Autodesk Inventor part; units mm, degrees
ref_plane "YZ Plane" through (0, 0, 0) normal (1, 0, 0) x (0, 1, 0)
ref_plane "XZ Plane" through (0, 0, 0) normal (0, 1, 0) x (-1, 0, 0)
ref_plane "XY Plane" through (0, 0, 0) normal (0, 0, 1) x (1, 0, 0)
sketch "Sketch1" plane through (0, 0, 0) normal (0, 0, 1) x (1, 0, 0)
  line L0 (-9.4319, 10.8445) -> (26.5681, 10.8445)
  line L1 (26.5681, 10.8445) -> (26.5681, -46.1555)
  line L2 (26.5681, -46.1555) -> (-9.4319, -46.1555)
  line L3 (-9.4319, -46.1555) -> (-9.4319, 10.8445)
  point P0 (0, 0)
  dimension "d0" = 36
  dimension "d1" = 57
extrude "Extrusion1" add sketch "Sketch1" along normal blind 3
sketch "Sketch2" plane through (-9.4319, 10.8445, 0) normal (0, 1, 0) x (1, 0, 0)
  line L0 (0, 0) -> (36, 0) construction
  line L1 (0, -3) -> (0, -22.268)
  line L2 (36, -3) -> (36, -22.268)
  line L3 (18, 0) -> (18, -6.949) construction
  arc A0 (36, -22.268) -> (0, -22.268) centre (18, -25.1836) ccw
  line L4 (36, -3) -> (0, -3)
  line L5 (36, -3) -> (0, -3)
  point P0 (9.4319, 0)
  dimension "d4" = 22.268
  dimension "d5" = 6.949
extrude "Extrusion2" add sketch "Sketch2" against normal blind 3
sketch "Sketch3" plane through (-9.4319, -46.1555, 0) normal (0, -1, 0) x (1, 0, 0)
  line L0 (0, 0) -> (0, 22.268) construction
  line L1 (36, 0) -> (36, 22.268) construction
  arc A0 (36, 28.0992) -> (0, 28.0992) centre (18, 25.1836) ccw
  line L2 (0, 22.268) -> (0, 28.0992)
  line L3 (36, 22.268) -> (36, 28.0992)
  line L4 (0, 3) -> (36, 3)
  arc A1 (0, 22.268) -> (36, 22.268) centre (18, 25.1836) ccw construction
  line L5 (0, 3) -> (0, 22.268)
  line L6 (36, 3) -> (36, 22.268)
  line L7 (0, 3) -> (36, 3)
  point P0 (9.4319, 0)
extrude "Extrusion3" add sketch "Sketch3" against normal blind 3
sketch "Sketch4" plane through (-9.4319, -46.1555, 0) normal (0, -1, 0) x (1, 0, 0)
  line L0 (0, 0) -> (36, 0)
  line L1 (18, 0) -> (18, 17.95) construction
  line L2 (18, 17.95) -> (18, 24.95) construction
  circle A0 centre (18, 24.95) radius 7
  line L3 (7.486, 24.95) -> (5.236, 24.95) construction
  circle A1 centre (5.236, 24.95) radius 2.25
  circle A2 centre (30.764, 24.95) radius 2.25
  point P0 (9.4319, 0)
  dimension "d10" = 17.95
  dimension "d11" = 7
  dimension "d13" = 2.25
extrude "Extrusion4" cut sketch "Sketch4" against normal blind 3
sketch "Sketch5" plane through (-9.4319, 10.8445, 0) normal (0, 1, 0) x (1, 0, 0)
  line L0 (36, 0) -> (0, 0)
  line L1 (36, 0) -> (36, -28.0992)
  line L2 (0, 0) -> (36, 0)
  line L3 (36, 0) -> (36, -6.35)
  line L4 (36, -6.35) -> (0, -6.35)
  line L5 (0, -6.35) -> (0, 0)
  point P0 (9.4319, 0)
  dimension "d17" = 6.35
extrude "Extrusion5" add sketch "Sketch5" along normal blind 25.7
sketch "Sketch6" plane through (-9.4319, 36.5445, 0) normal (0, 1, 0) x (1, 0, 0)
  line L0 (43.62, 0) -> (-7.62, 0)
  line L1 (-7.62, 0) -> (-7.62, -46.7504)
  line L2 (-7.62, -46.7504) -> (43.62, -46.7504)
  line L3 (43.62, -46.7504) -> (43.62, 0)
  line L4 (36, 0) -> (36, -28.0992)
  line L5 (0, 0) -> (0, -28.0992)
  dimension "d22" = 7.62
  dimension "d23" = 7.62
extrude "Extrusion6" add sketch "Sketch6" along normal blind 3
properties part number "motor connector"
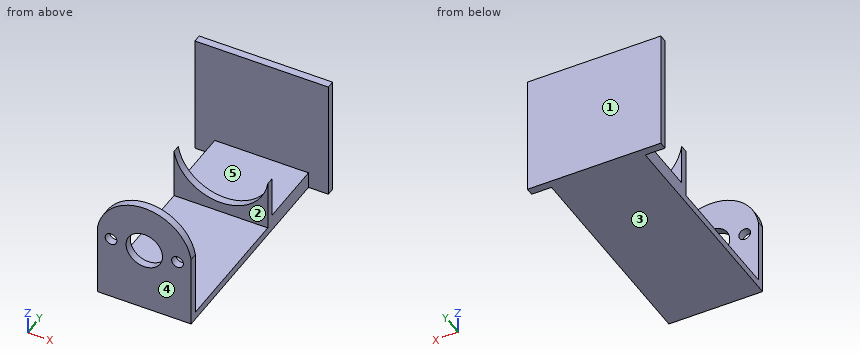
The listing builds one solid part. Answer for the finished solid, in the listing's coordinates (mm). Face numbers are marked on the shaded views. A direction names the side the tool comes from. Round coordinates to 2 decimals unless told otherwise and drop trailing zeros. Order: outer loops, then holes, each group sorted by start corner. A loop starts at its lowest first (then second) coordinate and runs counter-clockwise, first axis right, second up. Notation, with made-up numbers: (-10, 7) -> (41, 7) arc R18 ccw to (41, 24) -> close; hole circle Ø5 at (3, 63.25). An arc over 180 degrees is marked (long way). Put each result on its own line as item: value.
Q1. Consider line 1 along Y through (x, z) = (20, 7.5); line 2 along Y through (x, z) = (-1, 39.5); line 3 along X through (y, z) = (-44, 24). Determine where each line is inside the solid, lowest interval first.
Results list:
line 1: -46.16 to -43.16, 7.84 to 10.84, 36.54 to 39.54
line 2: -46.16 to -43.16, 36.54 to 39.54
line 3: -9.43 to -6.24, -2.16 to 1.63, 15.5 to 19.29, 23.37 to 26.57
Q2. Section C-C, the plane x = 6 is taken. Write down the section's boundary in (y, z).
Results list:
outline: (-46.16, 0) -> (39.54, 0) -> (39.54, 46.75) -> (36.54, 46.75) -> (36.54, 6.35) -> (10.84, 6.35) -> (10.84, 7.13) -> (7.84, 7.13) -> (7.84, 3) -> (-43.16, 3) -> (-43.16, 18.44) -> (-46.16, 18.44) -> close; (-46.16, 31.46) -> (-43.16, 31.46) -> (-43.16, 43.24) -> (-46.16, 43.24) -> close
Q3. Each of these flat-tipped pins is pushed along its axis until it touches: P1, Ø8, axis at x = 5, y = 28.5, coming from the +Z side; P2, Ø12, axis at y = -26.5, z = 8.5, coming from the +X side; P3, Ø4, axis at x = -4.2, z = 24.95, coming from the -Y side. Where does it stop, or does it pass through?
Results list:
P1: z = 6.35
P2: x = 26.57
P3: y = 36.54
Q4. Section A-A, the plane z = 24.95 is taken. Write down the section's boundary in (x, y), and give its area (3 significant figures).
Results list:
outline: (-17.05, 36.54) -> (34.19, 36.54) -> (34.19, 39.54) -> (-17.05, 39.54) -> close; (-9.43, -46.16) -> (-6.45, -46.16) -> (-6.45, -43.16) -> (-9.43, -43.16) -> close; (-1.95, -46.16) -> (1.57, -46.16) -> (1.57, -43.16) -> (-1.95, -43.16) -> close; (15.57, -46.16) -> (19.08, -46.16) -> (19.08, -43.16) -> (15.57, -43.16) -> close; (23.58, -46.16) -> (26.57, -46.16) -> (26.57, -43.16) -> (23.58, -43.16) -> close
area: 193 mm^2
Q5. Section D-D, the plane z = 16 is taken. Write down the section's boundary in (x, y), and give its area (3 significant figures).
Results list:
outline: (-17.05, 36.54) -> (34.19, 36.54) -> (34.19, 39.54) -> (-17.05, 39.54) -> close; (-9.43, -46.16) -> (26.57, -46.16) -> (26.57, -43.16) -> (-9.43, -43.16) -> close; (-9.43, 7.84) -> (-7.19, 7.84) -> (-7.19, 10.84) -> (-9.43, 10.84) -> close; (24.32, 7.84) -> (26.57, 7.84) -> (26.57, 10.84) -> (24.32, 10.84) -> close
area: 275 mm^2
Q6. Determine the mould class of the marked faces 3, 4 and 5 for opening direction Y: pulls with the +Y half, pulls with the -Y half, needs draft (parallel to the pull), parting line crosses it, or undercut.
Results list:
face 3: needs draft
face 4: pulls with the -Y half
face 5: undercut
Q7. Section B-B, the plane z = 42 is taken. Write down the section's boundary in (x, y).
Results list:
outline: (-17.05, 36.54) -> (34.19, 36.54) -> (34.19, 39.54) -> (-17.05, 39.54) -> close; (1.52, -46.16) -> (15.62, -46.16) -> (15.62, -43.16) -> (1.52, -43.16) -> close
Q8. Which of the six approach directions +Z, -Z, +X, -X, +Y, -Y give full straight-line access (tool end or side, diameter ignored) to the marked faces 1 and 2?
Results list:
face 1: +Z, -Z, +X, -X, +Y
face 2: +Z, +X, -X
